For this review, take the finished solid that the model builds, in its own axes (mm). Face numbers are marked on the shaded views. A direction names the side the tool comes from. Give positions to 0.01 mm unless a question says otherwise; leave off trailing zeros. Loops run counter-clockwise (first coordinate to the right, second up) from the corner with the lowest first, then second, coordinate; pieces in that order, holes last. Notation, with made-up numbers: M 82,-30.75 L 121,-30.75 A9 ccw 121,-15.75 Z; hole C 52,-10 d5. An arc over 180 degrees is marked long. Use CSV: the item, a comma, the result in double quotes. Start each with the question number.
1. Take a section at C-C, the plane x = 25.5. Write out the cut boundary in (y, z).
2. Tool access review of the marked faces 4 and 5: name each direction out of +Z, -Z, +X, -X, +Y, -Y from which nothing blocks a thin tool from reaching the whole face with its end or side.
3. Insertion check: P1, Ø15, axis at x = 29, y = 22, coming from the -Z side. The pin has a flat end and moves straight along its axis. Give the tip position at first contact, or say it passes through.
4. Take a section at B-B, the plane y = 13.5. Write out the cut boundary in (x, z), and give its area (3 significant figures).
5. Take a section at A-A, the plane z = 7.25. Write out the cut boundary in (x, y).
6. The part is to be moulded in two halves that separate along Y. For the marked faces 1, 2 and 3, say which applies: pulls with the +Y half, pulls with the -Y half, needs draft (parallel to the pull), parting line crosses it, or undercut.
7. To check wall thickness, follow line 1 (Y direction, x = 40.5, z = 12.25); line 2 (X direction, y = 12, z = 19.25); line 3 (Z direction, x = 7, y = 47.5). State the ranges of each line that lie inside material, in increasing order. Write a range as [from, to].
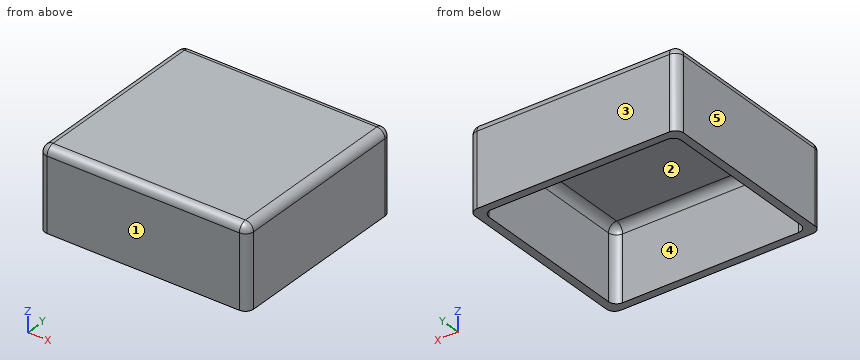
from build123d import *

# Parameters (mm, degrees)
F0_W     = 65.2412325144
F0_H     = 59.8419681191
F1_DEPTH = 25.4
F2_R     = 2.54
F3_T     = 2.54
F4_R     = 2.54


# Not quite as in the source:
# - a shell that OpenCascade refuses in one call is made with other operations: the cavity is built on its own and cut out


with BuildPart() as f1:
    # F0 (on Top) → F1 (new body)
    with BuildSketch(Plane.XY):
        with Locations((32.6206162572, 29.9209840596)):
            Rectangle(F0_W, F0_H)
    extrude(amount=F1_DEPTH)

    # F2
    f2_edges = [f1.edges().sort_by_distance(p)[0] for p in [
        (32.620616, 0, 25.4),
        (65.241233, 29.920984, 25.4),
        (32.620616, 59.841968, 25.4),
        (0, 29.920984, 25.4),
        (65.241233, 0, 12.7),
        (0, 0, 12.7),
        (65.241233, 59.841968, 12.7),
        (0, 59.841968, 12.7),
    ]]
    fillet(f2_edges, radius=F2_R)

    # F3: shell of thickness 2.54, made by hand


with BuildPart() as f3_core1:
    # F3_t2: copy of F1
    add(f1.part)

    # the walls: a layer under each face that stays
    f3_faces = [f3_core1.faces().sort_by_distance(p)[0] for p in [
        (0, 29.9209840596, 11.43),
        (32.6206162572, 59.8419681191, 11.43),
        (32.6206162572, 0, 11.43),
        (65.2412325144, 29.9209840596, 11.43),
        (32.6206162572, 29.9209840596, 25.4),
    ]]
    thicken(f3_faces, amount=-F3_T, mode=Mode.SUBTRACT)


with BuildPart() as f1_1:
    add(f1.part)

    # what is left inside the walls is the cavity
    f3_cavity = [f3_core1.part.solids().sort_by_distance(p)[0] for p in [
        (32.620616, 20.793989, 0.0254),
    ]]
    add(f3_cavity, mode=Mode.SUBTRACT)

    # F4
    f4_edges = [f1_1.edges().sort_by_distance(p)[0] for p in [
        (32.620616, 2.54, 22.86),
        (2.54, 29.920984, 22.86),
        (62.701233, 29.920984, 22.86),
        (32.620616, 57.301968, 22.86),
        (62.701233, 57.301968, 11.43),
        (2.54, 57.301968, 11.43),
        (2.54, 2.54, 11.43),
        (62.701233, 2.54, 11.43),
    ]]
    fillet(f4_edges, radius=F4_R)


solid = f1_1.part
Result set:
1,outline,"M 0,0 L 2.54,0 L 2.54,20.32 A2.54 cw 5.08,22.86 L 54.76,22.86 A2.54 cw 57.3,20.32 L 57.3,0 L 59.84,0 L 59.84,22.86 A2.54 ccw 57.3,25.4 L 2.54,25.4 A2.54 ccw 0,22.86 Z"
2,face 4,"-Z"
2,face 5,"+Z, -Z, -X, +Y, -Y"
3,P1,"z = 22.86"
4,outline,"M 0,0 L 2.54,0 L 2.54,20.32 A2.54 cw 5.08,22.86 L 60.16,22.86 A2.54 cw 62.7,20.32 L 62.7,0 L 65.24,0 L 65.24,22.86 A2.54 ccw 62.7,25.4 L 2.54,25.4 A2.54 ccw 0,22.86 Z"
4,area,"282 mm2"
5,outline,"M 0,2.54 A2.54 ccw 2.54,0 L 62.7,0 A2.54 ccw 65.24,2.54 L 65.24,57.3 A2.54 ccw 62.7,59.84 L 2.54,59.84 A2.54 ccw 0,57.3 Z; hole M 2.54,5.08 A2.54 ccw 5.08,2.54 L 60.16,2.54 A2.54 ccw 62.7,5.08 L 62.7,54.76 A2.54 ccw 60.16,57.3 L 5.08,57.3 A2.54 ccw 2.54,54.76 Z"
6,face 1,"pulls with the -Y half"
6,face 2,"undercut"
6,face 3,"pulls with the +Y half"
7,line 1,"[0, 2.54], [57.3, 59.84]"
7,line 2,"[0, 2.54], [62.7, 65.24]"
7,line 3,"[22.86, 25.4]"
